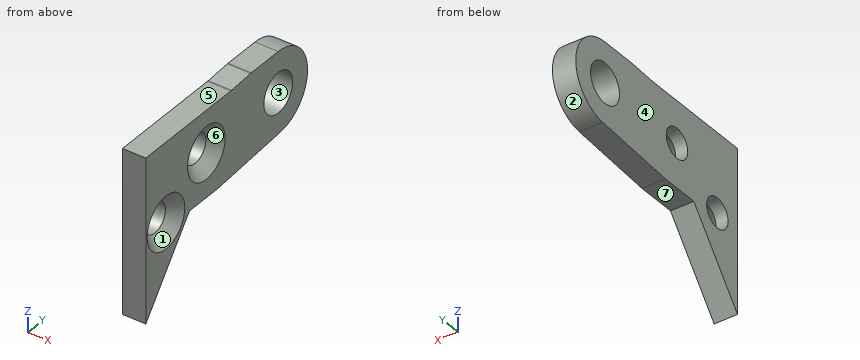
```python
from build123d import *

# Parameters (mm, degrees)
SKETCH1_R           = 2.15
BOSS_EXTRUDE1_DEPTH = 1.25
SKETCH3_R           = 1.6
CUT_EXTRUDE1_DEPTH  = 26.195485707
CHAMFER1_SIZE       = 1.2


with BuildPart() as part:
    # Sketch1 → Boss-Extrude1 (new, symmetric)
    with BuildSketch(Plane(origin=(0, 0, 0), x_dir=(0, 0, -1), z_dir=(1, 0, 0))):
        with BuildLine():
            Line((-4.35, 0), (-4.35, -4))
            ThreePointArc((-4.35, -4), (-4.349140426, -4.050773847), (-4.346562689, -4.101489502))
            Line((-4.346562689, -4.101489502), (-4.153437311, -6.949313458))
            ThreePointArc((-4.153437311, -6.949313458), (-4.150859574, -7.000029113), (-4.15, -7.050802959))
            Line((-4.15, -7.050802959), (-4.15, -20.2))
            Line((-4.15, -20.2), (14.85, -20.2))
            Line((14.85, -20.2), (5.393870957, -12.812062296))
            Line((5.393870957, -12.812062296), (4.33601498, 0.348531342))
            ThreePointArc((4.33601498, 0.348531342), (-0.174405904, 4.346502339), (-4.35, 0))
        make_face()
        Circle(SKETCH1_R, mode=Mode.SUBTRACT)
    extrude(amount=BOSS_EXTRUDE1_DEPTH, both=True)

    # Sketch3 → Cut-Extrude1 (cut, through all)
    with BuildSketch(Plane(origin=(1.25, 0, 0), x_dir=(0, 0, -1), z_dir=(1, 0, 0))):
        with Locations((0.35, -10.7)):
            Circle(SKETCH3_R)
        with Locations((4.35, -16.7)):
            Circle(SKETCH3_R)
        Polygon((-4.15, -20.2), (14.85, -20.2), (5.393870957, -12.812062296), (5.086040219, -8.982396127), (5.086040219, -13.206067673), (13.397894561, -19.7), (-4.15, -19.7), align=None)
    extrude(amount=-CUT_EXTRUDE1_DEPTH, mode=Mode.SUBTRACT)

    # Chamfer1
    chamfer1_edges = [part.edges().sort_by_distance(p)[0] for p in [
        (1.25, -16.7, -2.75),
        (1.25, -10.7, 1.25),
    ]]
    chamfer(chamfer1_edges, length=CHAMFER1_SIZE)


solid = part.part
```
Build history of the part. All positions in model axes, mm. Face numbers are marked on the shaded views. A direction names the side the tool comes from. Round coordinates to 2 decimals unless told otherwise and drop trailing zeros. Loops run counter-clockwise (first coordinate to the right, second up) from the corner with the lowest first, then second, coordinate; pieces in that order, holes last.
Item 1: Saw through at D-D (y = -10.7). List the corners of the cut face in (x, z).
Item 2: Two-plate mould, pull along Y, no slides. Class the marked faces 1, 2, 3 and 4: released by +Y, released by -Y, zero draft, split by the parting line, or undercut.
Item 3: Pin check, flat tips, straight feed: P1, Ø3, axis at y = -16.7, z = -4.35, coming from the -X side; P2, Ø1, axis at x = -1, z = -7.5, coming from the +Y side; P3, Ø0.8, axis at x = 0, y = -15.5, coming from the +Z side. Stop position of each tip, or through.
Item 4: Saw through at A-A (x = -0.75). List the corners of the cut face in (y, z).
Item 5: Saw through at B-B (y = -0.25). List the corners of the cut face in (x, z).
Item 6: Drill centre lines: line 1 along Y through (x, z) = (0.2, 0); line 2 along Y through (x, z) = (-0.9, -0.35); line 3 along Z through (x, y) = (-0.3, -9.25). Where is each one in solid material? Low to high.
Item 7: Saw through at C-C (x = 0.4). List the corners of the cut face in (y, z), then the cut area to 3 significant figures.
Item 8: Which spindle directions (+Z, -Z, +X, -X, +Y, -Y) get a long thin tool onto all of the face, cutting with end or side? Do the marked faces 5, 6 and 7. Say none if no direction does.
Worked answers:
1. outline: (-1.25, -5.09) - (1.25, -5.09) - (1.25, -3.15) - (0.05, -1.95) - (-1.25, -1.95) - close; (-1.25, 1.25) - (0.05, 1.25) - (1.25, 2.45) - (1.25, 4.15) - (-1.25, 4.15) - close
2. face 1: undercut
2. face 2: released by +Y
2. face 3: undercut
2. face 4: zero draft
3. P1: passes through
3. P2: stops at y = -14.7
3. P3: stops at z = 4.15
4. outline: (-19.7, -13.4) - (-13.21, -5.09) - (-8.98, -5.09) - (0.35, -4.34) arc R4.35 ccw to (0, 4.35) - (-4, 4.35) arc R1.5 ccw to (-4.1, 4.35) - (-6.95, 4.15) arc R1.5 cw to (-7.05, 4.15) - (-19.7, 4.15) - close; hole circle Ø3.2 at (-16.7, -4.35); hole circle Ø3.2 at (-10.7, -0.35); hole circle Ø4.3 at (0, 0)
5. outline: (-1.25, -4.38) - (1.25, -4.38) - (1.25, -2.14) - (-1.25, -2.14) - close; (-1.25, 2.14) - (1.25, 2.14) - (1.25, 4.35) - (-1.25, 4.35) - close
6. line 1: y = -19.7 to -12.41, -8.99 to -2.15, 2.15 to 4.35
6. line 2: y = -19.7 to -12.3, -9.1 to -2.12, 2.12 to 4.34
6. line 3: z = -5.09 to -1.03, 0.33 to 4.15
7. outline: (-19.7, -13.4) - (-13.21, -5.09) - (-8.98, -5.09) - (0.35, -4.34) arc R4.35 ccw to (0, 4.35) - (-4, 4.35) arc R1.5 ccw to (-4.1, 4.35) - (-6.95, 4.15) arc R1.5 cw to (-7.05, 4.15) - (-19.7, 4.15) - close; hole circle Ø3.9 at (-16.7, -4.35); hole circle Ø3.9 at (-10.7, -0.35); hole circle Ø4.3 at (0, 0)
7. area: 198 mm2
8. face 5: +Z, +X, -X, -Y
8. face 6: +X
8. face 7: -Z, +X, -X, +Y
